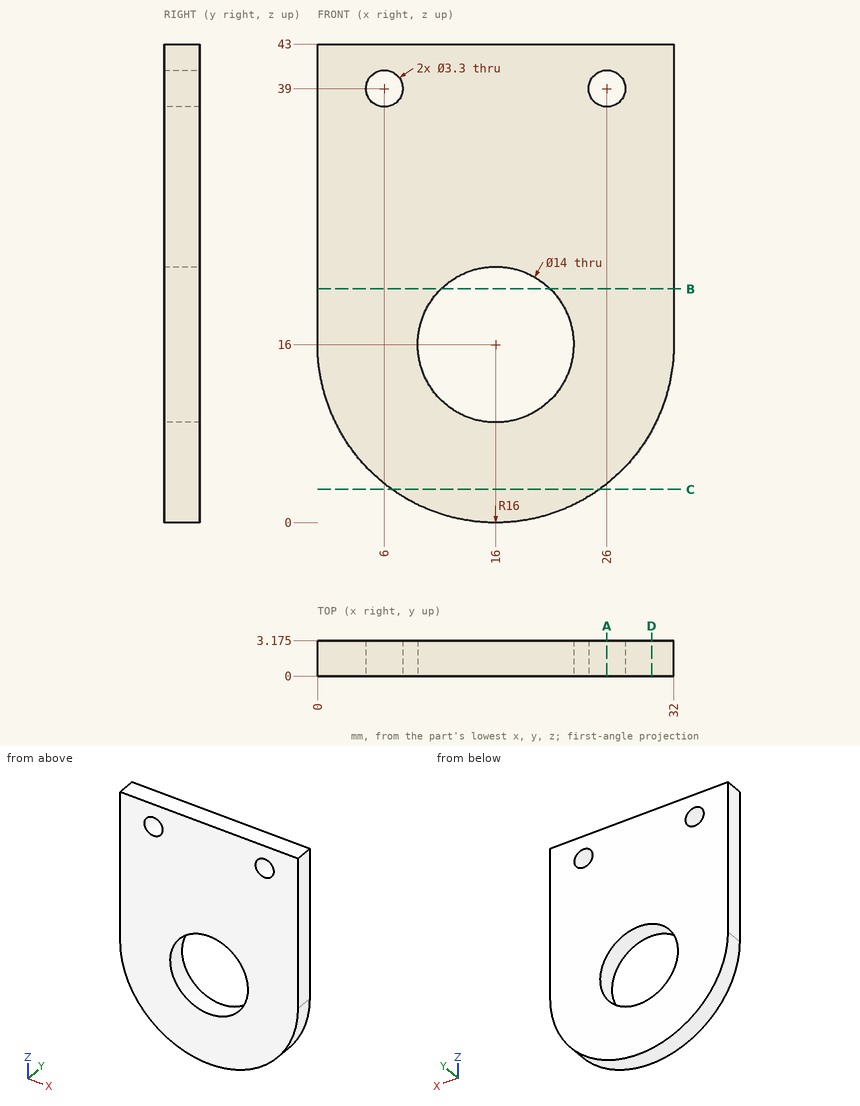
Job drawing, mm, ordinate dimensions from the low corner. One solid piece. Give positions to 0.01 mm unless a question says otherwise; leave off trailing zeros. Loops run counter-clockwise (first coordinate to the right, second up) from the corner with the lowest first, then second, coordinate; pieces in that order, holes last. Notation, with made-up numbers: M 28,78.5 L 34,78.5 A16 ccw 34,82.5 Z; hole C 6,-29 d3. An arc over 180 degrees is marked long. Answer in a Markdown table with one row per item. Add a question column.
Item 1: Band-saw the part on A-A on x = 26. Give the cut face in (y, z) (3 decimals), then the cut area to 3 significant figures.
Item 2: Band-saw the part on C-C on z = 3. Give the cut face in (x, y) (3 decimals), then the cut area to 3 significant figures.
Item 3: Probe probe 1 along X at (y, z) = (2.1, 39); probe 2 along X at (y, z) = (0.7, 16); probe 3 along Z at (x, y) = (11.5, 2.4). List the from-to ranges inside material, lowest first.
Item 4: Band-saw the part on B-B on z = 21. Give the cut face in (x, y) (3 decimals).
Item 5: Band-saw the part on D-D on x = 30. Give the cut face in (y, z) (3 decimals), then the cut area to 3 significant figures.
Reply:
| question | item | result |
|---|---|---|
| 1 | outline | M 0,3.51 L 3.175,3.51 L 3.175,37.35 L 0,37.35 Z; M 0,40.65 L 3.175,40.65 L 3.175,43 L 0,43 Z |
| 1 | area | 115 mm^2 |
| 2 | outline | M 6.673,0 L 25.327,0 L 25.327,3.175 L 6.673,3.175 Z |
| 2 | area | 59.2 mm^2 |
| 3 | probe 1 | x = 0 to 4.35, 7.65 to 24.35, 27.65 to 32 |
| 3 | probe 2 | x = 0 to 9, 23 to 32 |
| 3 | probe 3 | z = 0.65 to 10.64, 21.36 to 43 |
| 4 | outline | M 0,0 L 11.101,0 L 11.101,3.175 L 0,3.175 Z; M 20.899,0 L 32,0 L 32,3.175 L 20.899,3.175 Z |
| 5 | outline | M 0,8.254 L 3.175,8.254 L 3.175,43 L 0,43 Z |
| 5 | area | 110 mm^2 |
